from build123d import *

# Parameters (mm, degrees)
F0_R     = 11
F1_DEPTH = 7.62
F2_SIZE  = 3.80999


# Not quite as in the source:
# - a fillet or chamfer is up to 0.001 mm smaller than in the source, because OpenCascade refuses the exact size


with BuildPart() as f1:
    # F0 (on Top) → F1 (new body)
    with BuildSketch(Plane.XY):
        with BuildLine():
            Line((6.35, 25.4), (-6.35, 25.4))
            ThreePointArc((-6.35, 25.4), (-11.9296158184, 11.9296158184), (-25.4, 6.35))
            Line((-25.4, 6.35), (-25.4, -6.35))
            ThreePointArc((-25.4, -6.35), (-11.9296158184, -11.9296158184), (-6.35, -25.4))
            Line((-6.35, -25.4), (6.35, -25.4))
            ThreePointArc((6.35, -25.4), (11.9296158184, -11.9296158184), (25.4, -6.35))
            Line((25.4, -6.35), (25.4, 6.35))
            ThreePointArc((25.4, 6.35), (11.9296158184, 11.9296158184), (6.35, 25.4))
        make_face()
        Circle(F0_R, mode=Mode.SUBTRACT)
    extrude(amount=F1_DEPTH)

    # F2 (size 3.81 in the source; OpenCascade refuses exactly that, so slightly less here)
    f2_edges = [f1.edges().sort_by_distance(p)[0] for p in [
        (11.929616, 11.929616, 7.62),
        (-11.929616, 11.929616, 7.62),
        (0, 25.4, 7.62),
        (25.4, 0, 7.62),
        (11.929616, -11.929616, 7.62),
        (0, -25.4, 7.62),
        (-11.929616, -11.929616, 7.62),
        (-25.4, 0, 7.62),
        (-11.929616, 11.929616, 0),
        (0, 25.4, 0),
        (11.929616, 11.929616, 0),
        (11.929616, -11.929616, 0),
        (25.4, 0, 0),
        (-11.929616, -11.929616, 0),
        (0, -25.4, 0),
        (-25.4, 0, 0),
    ]]
    chamfer(f2_edges, length=F2_SIZE)


solid = f1.part
Can you work these out from the model? Positions are in its coordinate system, mm. Coordinates: 2 decimals unless noted, no trailing zeros. Order: outer loops, then holes, each group sorted by start corner. A loop starts at its lowest first (then second) coordinate and runs counter-clockwise, first axis right, second up. Notation, with made-up numbers: M 30.5,65 L 66.5,65 A23 ccw 66.5,84 Z; hole C 30,44 d5. An arc over 180 degrees is marked long. Write item = value, one per line.
(1) For pin 1 Ø12 at (x, y) = (17.5, -6) entering from +Z; pin 2 Ø2 at (y, z) = (-12, 1.5) entering from +X; pin 3 Ø1 at (y, z) = (-20, 2.5) entering from -X, each with a flat end and sliding along its axis, tell me the tip position at first contact or that it passes through.
Results are:
pin_1 = 7.62
pin_2 = 10.34
pin_3 = -6.31
(2) Suppose I cut it at C-C on z = 4.75. Please give me the cut outline in (x, y).
Results are:
outline = M -24.46,-5.43 A19.99 cw -5.43,-24.46 L 5.43,-24.46 A19.99 cw 24.46,-5.43 L 24.46,5.43 A19.99 cw 5.43,24.46 L -5.43,24.46 A19.99 cw -24.46,5.43 Z; hole C 0,0 d22
(3) Suppose I cut it at D-D on z = 2. Please give me the cut outline in (x, y), plus the area to 3 significant figures.
Results are:
outline = M -23.59,-4.62 A20.86 cw -4.62,-23.59 L 4.62,-23.59 A20.86 cw 23.59,-4.62 L 23.59,4.62 A20.86 cw 4.62,23.59 L -4.62,23.59 A20.86 cw -23.59,4.62 Z; hole C 0,0 d22
area = 767 mm2
(4) I need wall thicknesses on line 1 along X through (y, z) = (7, 1.5); line 2 along X through (y, z) = (-7, 2.5); line 3 along Y through (x, z) = (-8, 1.25). Which ranges of each line are inside material? Lowest first, please. Write a range as [from, to].
Results are:
line_1 = [-14.55, -8.49], [8.49, 14.55]
line_2 = [-16.68, -8.49], [8.49, 16.68]
line_3 = [-12.58, -7.55], [7.55, 12.58]
